from build123d import *
from OCP.BRepFilletAPI import BRepFilletAPI_MakeChamfer

# Parameters (mm, degrees)
BOSS_EXTRUDE1_DEPTH = 6.35
CHAMFER1_SIZE       = 12.7
CHAMFER1_SIZE2      = 3.048
CHAMFER2_SIZE       = 3.048
CHAMFER2_SIZE2      = 12.7


with BuildPart() as part:
    # Sketch2 → Boss-Extrude1 (new body)
    with BuildSketch(Plane.XY):
        Polygon((0, 0), (0, 393.7), (152.414038874, -16.129), (152.414038874, -92.329), align=None)
    extrude(amount=BOSS_EXTRUDE1_DEPTH)

    # Chamfer1
    chamfer1_edges = [part.edges().sort_by_distance(p)[0] for p in [
        (76.207019437, 188.7855, 0),
        (76.207019437, -46.1645, 0),
    ]]
    chamfer1_side = [part.faces().sort_by_distance(p)[0] for p in [
        (59.04327632, 99.585162162, 0),
    ]]
    chamfer(chamfer1_edges, length=CHAMFER1_SIZE, length2=CHAMFER1_SIZE2, reference=chamfer1_side[0])

    # Chamfer2: one chamfer whose edges measure the first distance from different faces: ONE call of the kernel's chamfer builder (chamfer() names one face for all edges)
    chamfer2_edges_1 = [part.edges().sort_by_distance(p)[0] for p in [
        (76.207019437, 188.7855, 6.35),
    ]]
    chamfer2_side_1 = [part.faces().sort_by_distance(p)[0] for p in [
        (76.207019437, 188.7855, 4.699),
    ]]
    chamfer2_edges_2 = [part.edges().sort_by_distance(p)[0] for p in [
        (76.207019437, -46.1645, 6.35),
    ]]
    chamfer2_side_2 = [part.faces().sort_by_distance(p)[0] for p in [
        (76.207019437, -46.1645, 4.699),
    ]]
    chamfer2 = BRepFilletAPI_MakeChamfer(part.part.solid().wrapped)
    for e in chamfer2_edges_1:
        chamfer2.Add(CHAMFER2_SIZE, CHAMFER2_SIZE2, e.wrapped, chamfer2_side_1[0].wrapped)  # the first distance lies on this face
    for e in chamfer2_edges_2:
        chamfer2.Add(CHAMFER2_SIZE, CHAMFER2_SIZE2, e.wrapped, chamfer2_side_2[0].wrapped)  # the first distance lies on this face
    add(Compound.cast(chamfer2.Shape()), mode=Mode.REPLACE)


solid = part.part
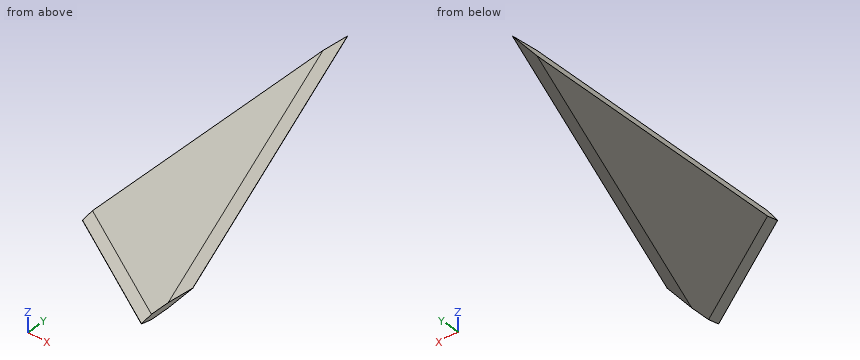
Geometry: final body of the model. Coordinates: model frame, mm. Give positions to 0.01 mm unless a question says otherwise; leave off trailing zeros. Loops run counter-clockwise (first coordinate to the right, second up) from the corner with the lowest first, then second, coordinate; pieces in that order, holes last. Notation, with made-up numbers: (-23.5, -31.5) - (33.5, -31.5) arc R37 cw to (33.5, 5.5) - close; hole circle Ø6 at (-38, 5). An arc over 180 degrees is marked (long way). Answer as CSV lines item,"result". Start each with the question number.
1. Section D-D, the plane x = 138. Return loops of the section in (y, z), plus the area to 3 significant figures.
2. Section C-C, the plane z = 1.25. Return loops of the section in (x, y), plus the area to 3 significant figures.
3. Section A-A, the plane x = 109.5. Return loops of the section in (y, z).
4. Section B-B, the plane y = 269. Return loops of the section in (x, z), plus the area to 3 significant figures.
5. Ray query, L1, parallel to Z at x = 132, y = 16.5; L2, parallel to Z at x = 115, y = 57. Return the intervals inside material, ascending.
6. Pin query (flat end, axial travel): P1, Ø1.5, axis at x = 51, z = 2.5, coming from the -Y side. Return the tip coordinate at first contact, or that it passes through.
Answers:
1,outline,"(-83.6, 3.05) - (-68.75, 0) - (-13.81, 0) - (22.63, 3.05) - (22.63, 3.3) - (-13.81, 6.35) - (-68.75, 6.35) - (-83.6, 3.3) - close"
1,area,"518 mm2"
2,outline,"(0, 8.76) - (152.41, -83.57) - (152.41, -37.62) - (0, 372.21) - close"
2,area,"31,200 mm2"
3,outline,"(-66.33, 3.05) - (-51.48, 0) - (62.83, 0) - (99.26, 3.05) - (99.26, 3.3) - (62.83, 6.35) - (-51.48, 6.35) - (-66.33, 3.3) - close"
4,outline,"(0, 0) - (32.83, 0) - (46.38, 3.05) - (46.38, 3.3) - (32.83, 6.35) - (0, 6.35) - close"
4,area,"253 mm2"
5,L1,"z = 1.19 to 5.16"
5,L2,"z = 0.75 to 5.6"
6,P1,"stops at y = -31.2"
